Solid Edge part; units mm, degrees
sketch "Sketch1" plane through (0, 0, 0) normal (0, 0, 1) x (1, 0, 0)
  circle A0 centre (0, 0) radius 125
extrude "Protrusion1" add sketch "Sketch1" against normal blind 6
sketch "Sketch2" plane through (0, 0, 0) normal (0, 0, 1) x (1, 0, 0)
  circle A0 centre (0, 0) radius 115
extrude "Cutout1" cut sketch "Sketch2" against normal through all
sketch "Sketch3" plane through (0, 0, 0) normal (0, 0, 1) x (1, 0, 0)
  line L0 (-5, 117) -> (5, 117)
  line L1 (5, 117) -> (5, 123)
  line L2 (5, 123) -> (-5, 123)
  line L3 (-5, 123) -> (-5, 117)
  dimension "D1" = 5
  dimension "D2" = 5
extrude "Cutout2" cut sketch "Sketch3" against normal through all
pattern_circular "Pattern1" count 4 over 360 about axis through (0, 0, 0) along (0, 0, -1) of "Cutout2"
properties material "Wood, Mahogany"
Verification items for the finished model (mm, model axes). A direction names the side the tool comes from. Give positions to 0.01 mm unless a question says otherwise; leave off trailing zeros. Loops run counter-clockwise (first coordinate to the right, second up) from the corner with the lowest first, then second, coordinate; pieces in that order, holes last. Notation, with made-up numbers: (-14.75, -17.5) - (39.25, -17.5) arc R25 ccw to (39.25, 13.5) - close; hole circle Ø9 at (49.25, 1.25). An arc over 180 degrees is marked (long way). Write each question's results on one line, items separated by ' | '.
1) Sectioned sample at D-D on x = -79. Record the boundary of the cut face in (y, z), plus the area to 3 significant figures.
Solution:
outline: (-96.87, -6) - (-83.57, -6) - (-83.57, 0) - (-96.87, 0) - close; (83.57, -6) - (96.87, -6) - (96.87, 0) - (83.57, 0) - close | area: 160 mm2
2) Material ranges on L1, parallel to Y at x = 0, z = -3.15; L2, parallel to X at y = -6.5, z = -4.55; L3, parallel to X at y = -75, z = -1.15, recorded low to high. Write a range as from..to.
Solution:
L1: -125..-123, -117..-115, 115..117, 123..125 | L2: -124.83..-114.82, 114.82..124.83 | L3: -100..-87.18, 87.18..100
3) Mould release check, pull along Y, two halves, no side actions. Record for faces 1 (the flat face through (55, -101.3, 0)), 2 (the flat face through (123, 0, -3)), 3 (the cylindrical face through (-124.88, 5.5, -2.96)): pulls with the +Y half, pulls with the -Y half, needs draft (parallel to the pull), parting line crosses it, or undercut.
Solution:
face 1: needs draft | face 2: undercut | face 3: parting line crosses it
4) Sectioned sample at B-B on x = 0. Record the boundary of the cut face in (y, z), plus the area to 3 significant figures.
Solution:
outline: (-125, -6) - (-123, -6) - (-123, 0) - (-125, 0) - close; (-117, -6) - (-115, -6) - (-115, 0) - (-117, 0) - close; (115, -6) - (117, -6) - (117, 0) - (115, 0) - close; (123, -6) - (125, -6) - (125, 0) - (123, 0) - close | area: 48.0 mm2
5) Tool access check on faces 4 (the flat face through (55, -101.3, -6)), 5 (the flat face through (117, 0, -3)). Record the directions out of +Z, -Z, +X, -X, +Y, -Y that give a thin tool (end or side, any length) a straight path to the whole face; none if there is none.
Solution:
face 4: -Z, +X, -X, +Y, -Y | face 5: +Z, -Z
6) Depth check by flat-ended pin: P1, Ø2, axis at x = 67.5, z = -3.5, coming from the +Y side; P2, Ø1.5, axis at y = -79.5, z = -3, coming from the -X side. Enter the tip coordinate at first touch or a pass-through.
Solution:
P1: y = 105.84 | P2: x = -97.07
7) Sectioned sample at A-A on z = -2.3. Record the boundary of the cut face in (x, y).
Solution:
outline: circle Ø250 at (0, 0); hole (-123, -5) - (-117, -5) - (-117, 5) - (-123, 5) - close; hole circle Ø230 at (0, 0); hole (-5, -123) - (5, -123) - (5, -117) - (-5, -117) - close; hole (-5, 117) - (5, 117) - (5, 123) - (-5, 123) - close; hole (117, -5) - (123, -5) - (123, 5) - (117, 5) - close
